Autodesk Inventor part; units mm, degrees
ref_plane "YZ Plane" through (0, 0, 0) normal (1, 0, 0) x (0, 1, 0)
ref_plane "XZ Plane" through (0, 0, 0) normal (0, 1, 0) x (-1, 0, 0)
ref_plane "XY Plane" through (0, 0, 0) normal (0, 0, 1) x (1, 0, 0)
sketch "Sketch1" plane through (0, 0, 0) normal (0, 0, 1) x (1, 0, 0)
  line L0 (-51.4052, 38.5707) -> (3.5948, 38.5707)
  line L1 (3.5948, 38.5707) -> (3.5948, -19.4293)
  line L2 (3.5948, -19.4293) -> (-51.4052, -19.4293)
  line L3 (-51.4052, -19.4293) -> (-51.4052, 38.5707)
  line L4 (-54.4052, 41.5707) -> (6.5948, 41.5707)
  line L5 (6.5948, 41.5707) -> (6.5948, -22.4293)
  line L6 (6.5948, -22.4293) -> (-54.4052, -22.4293)
  line L7 (-54.4052, -22.4293) -> (-54.4052, 41.5707)
  line L8 (-48.4052, 35.5707) -> (0.5948, 35.5707)
  line L9 (0.5948, 35.5707) -> (0.5948, -16.4293)
  line L10 (0.5948, -16.4293) -> (-48.4052, -16.4293)
  line L11 (-48.4052, -16.4293) -> (-48.4052, 35.5707)
  point P0 (0, 0)
  dimension "d0" = 55
  dimension "d1" = 58
  dimension "d2" = 3
  dimension "d3" = 3
  dimension "d4" = 3
  dimension "d5" = 3
  dimension "d6" = 3
  dimension "d7" = 3
  dimension "d8" = 3
  dimension "d9" = 3
extrude "Extrusion1" add sketch "Sketch1" along normal blind 2 contours L0 L1 L2 L3 | L4 L5 L6 L7
sketch "Sketch2" plane through (0, 0, 2) normal (0, 0, 1) x (1, 0, 0)
  line L0 (-54.4052, 41.5707) -> (-54.4052, -22.4293)
  line L1 (6.5948, 41.5707) -> (-54.4052, 41.5707)
  line L2 (6.5948, 41.5707) -> (6.5948, -22.4293)
  line L3 (-54.4052, -22.4293) -> (6.5948, -22.4293)
  point P0 (0, 0)
  point P1 (-51.4052, 38.5707)
  point P2 (3.5948, 38.5707)
  point P3 (3.5948, -19.4293)
  point P4 (-51.4052, -19.4293)
  dimension "d12" = 3
  dimension "d13" = 3
  dimension "d14" = 3
  dimension "d15" = 3
  dimension "d16" = 3
  dimension "d17" = 3
  dimension "d18" = 3
  dimension "d19" = 3
hole "Hole1" at (-51.4052, 38.5707, 2) at (3.5948, 38.5707, 2) at (3.5948, -19.4293, 2) at (-51.4052, -19.4293, 2) direction (0, 0, -1) diameter 3 depth 8 tip angle 118 countersink diameter 6 countersink angle 90
sketch "Sketch3" plane through (0, 0, 2) normal (0, 0, 1) x (1, 0, 0)
  line L0 (-48.4052, -16.4293) -> (-48.4052, 35.5707)
  line L1 (0.5948, 35.5707) -> (-48.4052, 35.5707)
  line L2 (0.5948, 35.5707) -> (0.5948, -16.4293)
  line L3 (-48.4052, -16.4293) -> (0.5948, -16.4293)
  line L4 (-48.4052, 33.5707) -> (-1.4052, -16.4293)
  line L5 (-1.4052, -16.4293) -> (0.5948, -16.4293)
  line L6 (0.5948, -16.4293) -> (0.5948, -14.4293)
  line L7 (0.5948, -14.4293) -> (-46.4052, 35.5707)
  line L8 (-48.4052, 35.5707) -> (-46.4052, 35.5707)
  line L9 (-48.4052, 35.5707) -> (-48.4052, 33.5707)
  line L10 (-48.4052, -14.4293) -> (-1.4052, 35.5707)
  line L11 (-1.4052, 35.5707) -> (0.5948, 35.5707)
  line L12 (0.5948, 33.5707) -> (-46.4052, -16.4293)
  line L13 (-46.4052, -16.4293) -> (-48.4052, -16.4293)
  line L14 (-48.4052, -16.4293) -> (-48.4052, -14.4293)
  point P0 (0, 0)
  point P1 (-46.4052, -16.4293)
  dimension "d27" = 2
  dimension "d28" = 2
  dimension "d29" = 2
  dimension "d30" = 2
  dimension "d31" = 2
  dimension "d32" = 2
  dimension "d33" = 2
  dimension "d34" = 2
extrude "Extrusion2" add sketch "Sketch3" against normal blind 2 contours L0 L10 L4 L12 L3 | L0 L1 L7 L10 L4 | L10 L7 L12 L4 | L4 L12 L7 L2 L3 | L10 L1 L2 L12 L7
chamfer "Chamfer1" distance 2 angle 45 8 edges at (-46.4052, 35.5707, 1) (-48.4052, 33.5707, 1) (0.5948, 33.5707, 1) (-1.4052, 35.5707, 1) (0.5948, -14.4293, 1) (-1.4052, -16.4293, 1) (-48.4052, -14.4293, 1) (-46.4052, -16.4293, 1)
properties part number "Mounting Plate"
The listing builds one solid part. Answer for the finished solid, in the listing's coordinates (mm). A direction names the side the tool comes from. Coordinates: 2 decimals unless noted, no trailing zeros. Loops run counter-clockwise (first coordinate to the right, second up) from the corner with the lowest first, then second, coordinate; pieces in that order, holes last. Notation, with made-up numbers: (-29.75, 18.5) -> (-8.75, 18.5) arc R28 ccw to (-8.75, 36.5) -> close; hole circle Ø7 at (-34, -27.75). An arc over 180 degrees is marked (long way). Write item = value, one per line. Start each with the question number.
1) A cutting plane is placed at C-C (y = -0.5). Give the vertices of the cut face in (x, z).
2) Straight lines are drawn through the part: line 1 (X direction, y = 29, z = 1.7); line 2 (X direction, y = -6.5, z = 1.75); line 3 (Y direction, x = -20, z = 0.35). For each, find the intervals that lie inside material, in ascending order. Write a range as from..to.
3) The mould has two halves that part along Y. Classify faces 1 (the face through (-24, 10, 0)), 2 (the face through (-0.1, -12.704, 1.014)): released by +Y, released by -Y, zero draft, split by the parting line, or undercut.
4) A cutting plane is placed at A-A (x = -14). Give the vertices of the cut face in (y, z).
5) A tool of negligible diameter and unlimited length cuts with its end or side. For faces 3 (the face through (-34.322, 22.717, 1.014)), 4 (the face through (6, 41, 2)), from which of +Z, -Z, +X, -X, +Y, -Y can it reach the whole face along a straight path? Write none if from no direction.
6) A cutting plane is placed at D-D (y = 33). Give the vertices of the cut face in (x, z), then the cut area to 3 significant figures.
7) Given pin 1 Ø1 at (x, y) = (-26.5, 3) entering from -Z, flat-ended and moving along its own axis, determine where the tip first touches the part or whether it passes through.
8) A cutting plane is placed at B-B (z = 1.35). Count the separate pieces of the cut face and the enclosed holes in it, then the cut area to 3 significant figures.
Responses:
q1.outline = (-54.41, 0) -> (-48.41, 0) -> (-48.41, 2) -> (-54.41, 2) -> close; (-35.31, 0) -> (-31.43, 0) -> (-31.43, 2) -> (-35.31, 2) -> close; (-16.38, 0) -> (-12.5, 0) -> (-12.5, 2) -> (-16.38, 2) -> close; (0.59, 0) -> (6.59, 0) -> (6.59, 2) -> (0.59, 2) -> close
q2.line_1 = -54.41..-48.41, -44.11..-40.23, -7.58..-3.7, 0.59..6.59
q2.line_2 = -54.41..-48.41, -40.95..-37.07, -10.74..-6.86, 0.59..6.59
q2.line_3 = -22.43..-16.43, 3.35..7.48, 11.66..15.79, 35.57..41.57
q3.face_1 = zero draft
q3.face_2 = undercut
q4.outline = (-22.43, 0) -> (-16.43, 0) -> (-16.43, 2) -> (-22.43, 2) -> close; (-3.03, 0) -> (1.1, 0) -> (1.1, 2) -> (-3.03, 2) -> close; (18.04, 0) -> (22.17, 0) -> (22.17, 2) -> (18.04, 2) -> close; (35.57, 0) -> (41.57, 0) -> (41.57, 2) -> (35.57, 2) -> close
q5.face_3 = +Z, -Z
q5.face_4 = +Z, +X, -X, +Y, -Y
q6.outline = (-54.41, 0) -> (-43.99, 0) -> (-43.99, 2) -> (-54.41, 2) -> close; (-3.82, 0) -> (6.59, 0) -> (6.59, 2) -> (-3.82, 2) -> close
q6.area = 41.7 mm²
q7.pin_1 = through
q8.separate_pieces = 1
q8.enclosed_holes = 8
q8.area = 1,690 mm²
